Check sheet for the modelled part. Datum: model origin and axes. Units: mm. A direction names the side the tool comes from. Round coordinates to 2 decimals unless told otherwise and drop trailing zeros. Order: outer loops, then holes, each group sorted by start corner. A loop starts at its lowest first (then second) coordinate and runs counter-clockwise, first axis right, second up.
(1) Tool access check on faces 5 (the cylindrical face through (-11.93, 10.55, 18.72)), 6 (the cylindrical face through (35.15, 3.45, 6.24)). Record the directions out of +Z, -Z, +X, -X, +Y, -Y that give a thin tool (end or side, any length) a straight path to the whole face; none if there is none.
(2) Sectioned sample at B-B, the plane y = 4.25. Enter the section's corners in (x, z).
(3) Sectioned sample at A-A, the plane x = 0. Enter the section's corners in (y, z), and give its area (3 significant figures).
(4) Depth check by flat-ended pin: pin 1 (5.5 mm diameter, centred on x = -28, z = 0, fed in from -Y); pin 2 (3 mm diameter, centred on x = -4, y = 3.5, fed in from -Z); pin 3 (10 mm diameter, centred on x = 27.5, z = -4.5, fed in from +Y); pin 4 (4 mm diameter, centred on y = 4.5, z = 15.5, fed in from -X). Enter the tip coordinate at first touch or a pass-through.
(5) Sectioned sample at D-D, the plane z = 0. Count the separate pieces of the cut face and the enclosed holes in it, and give its area (3 significant figures).
(6) Sectioned sample at C-C, the plane y = 9.5. Enter the section's corners in (x, z), and give its area (3 significant figures).
(7) Mould release check, pull along X, two halves, no side actions. Record for faces 1 (the flat face through (3, 14, -20)), 2 (the cylindrical face through (-16.88, 11.26, 5.32)), 3 (the cylindrical face through (-24.66, 3.45, -1.05)), 4 (the flat face through (-35.5, 3, 0)): released by +X, released by -X, zero draft, split by the parting line, or undercut.
(8) Thickness scan on probe 1 along X at (y, z) = (4, 0); probe 2 along Z at (x, y) = (0, 11.25); probe 3 along Z at (x, y) = (0, 9.25). Record the ranges inside material, lowest first.
```python
from build123d import *

# Parameters (mm, degrees)
SKETCH1_R           = 3.5
SKETCH1_R_2         = 8.5
BOSS_EXTRUDE1_DEPTH = 7


with BuildPart() as part:
    # Sketch1 → Boss-Extrude1 (new body)
    with BuildSketch(Plane(origin=(0, 0, 0), x_dir=(1, 0, 0), z_dir=(0, 1, 0))):
        with BuildLine():
            Line((19.915308817, 12.274508393), (34.194882732, 6.983577796))
            ThreePointArc((34.194882732, 6.983577796), (35.141609799, 6.250591667), (35.5, 5.108174376))
            Line((35.5, 5.108174376), (35.5, -5.108174376))
            ThreePointArc((35.5, -5.108174376), (35.141609799, -6.250591667), (34.194882732, -6.983577796))
            Line((34.194882732, -6.983577796), (19.915308817, -12.274508393))
            ThreePointArc((19.915308817, -12.274508393), (19.380803519, -12.572380491), (18.961376225, -13.017918868))
            ThreePointArc((18.961376225, -13.017918868), (0, -23), (-18.961376225, -13.017918868))
            ThreePointArc((-18.961376225, -13.017918868), (-19.380803519, -12.572380491), (-19.915308817, -12.274508393))
            Line((-19.915308817, -12.274508393), (-34.194882732, -6.983577796))
            ThreePointArc((-34.194882732, -6.983577796), (-35.141609799, -6.250591667), (-35.5, -5.108174376))
            Line((-35.5, -5.108174376), (-35.5, 5.108174376))
            ThreePointArc((-35.5, 5.108174376), (-35.141609799, 6.250591667), (-34.194882732, 6.983577796))
            Line((-34.194882732, 6.983577796), (-19.915308817, 12.274508393))
            ThreePointArc((-19.915308817, 12.274508393), (-19.380803519, 12.572380491), (-18.961376225, 13.017918868))
            ThreePointArc((-18.961376225, 13.017918868), (0, 23), (18.961376225, 13.017918868))
            ThreePointArc((18.961376225, 13.017918868), (19.380803519, 12.572380491), (19.915308817, 12.274508393))
        make_face()
        with Locations((28, 0)):
            Circle(SKETCH1_R, mode=Mode.SUBTRACT)
        with Locations((-28, 0)):
            Circle(SKETCH1_R, mode=Mode.SUBTRACT)
        Circle(SKETCH1_R_2, mode=Mode.SUBTRACT)
    extrude(amount=BOSS_EXTRUDE1_DEPTH)

    # Sketch2 → Revolve1 (revolve)
    with BuildSketch(Plane.XY):
        Polygon((-8.5, 15), (-8.5, 7), (-22.2, 7), (-22.2, 14), (-19.7, 14), (-19.7, 10.918286082), (-17.7, 10.918286082), (-17.7, 11.6), (-15.7, 11.6), (-15.7, 11), (-10.5, 11), (-10.5, 15), align=None)
    revolve(axis=Axis((0, 0, 0), (0, 1, 0)))


solid = part.part
```
Derived:
1. face 5: +Y
1. face 6: +Z, +X, +Y, -Y
2. outline: (-35.5, -5.11) arc R2 ccw to (-34.19, -6.98) - (-19.92, -12.27) arc R2 cw to (-18.96, -13.02) arc R23 ccw to (18.96, -13.02) arc R2 cw to (19.92, -12.27) - (34.19, -6.98) arc R2 ccw to (35.5, -5.11) - (35.5, 5.11) arc R2 ccw to (34.19, 6.98) - (19.92, 12.27) arc R2 cw to (18.96, 13.02) arc R23 ccw to (-18.96, 13.02) arc R2 cw to (-19.92, 12.27) - (-34.19, 6.98) arc R2 ccw to (-35.5, 5.11) - close; hole circle Ø7 at (-28, 0); hole circle Ø17 at (0, 0); hole circle Ø7 at (28, 0)
3. outline: (0, -23) - (7, -23) - (7, -22.2) - (14, -22.2) - (14, -19.7) - (10.92, -19.7) - (10.92, -17.7) - (11.6, -17.7) - (11.6, -15.7) - (11, -15.7) - (11, -10.5) - (15, -10.5) - (15, -8.5) - (0, -8.5) - close; (0, 8.5) - (15, 8.5) - (15, 10.5) - (11, 10.5) - (11, 15.7) - (11.6, 15.7) - (11.6, 17.7) - (10.92, 17.7) - (10.92, 19.7) - (14, 19.7) - (14, 22.2) - (7, 22.2) - (7, 23) - (0, 23) - close
3. area: 346 mm2
4. pin 1: passes through
4. pin 2: stops at z = -22.86
4. pin 3: stops at y = 7
4. pin 4: stops at x = -18.62
5. separate pieces: 4
5. enclosed holes: 0
5. area: 423 mm2
6. outline: circle Ø44.4 at (0, 0); hole circle Ø17 at (0, 0)
6. area: 1,320 mm2
7. face 1: zero draft
7. face 2: undercut
7. face 3: undercut
7. face 4: released by -X
8. probe 1: x = -35.5 to -31.5, -24.5 to -8.5, 8.5 to 24.5, 31.5 to 35.5
8. probe 2: z = -22.2 to -19.7, -17.7 to -15.7, -10.5 to -8.5, 8.5 to 10.5, 15.7 to 17.7, 19.7 to 22.2
8. probe 3: z = -22.2 to -8.5, 8.5 to 22.2
